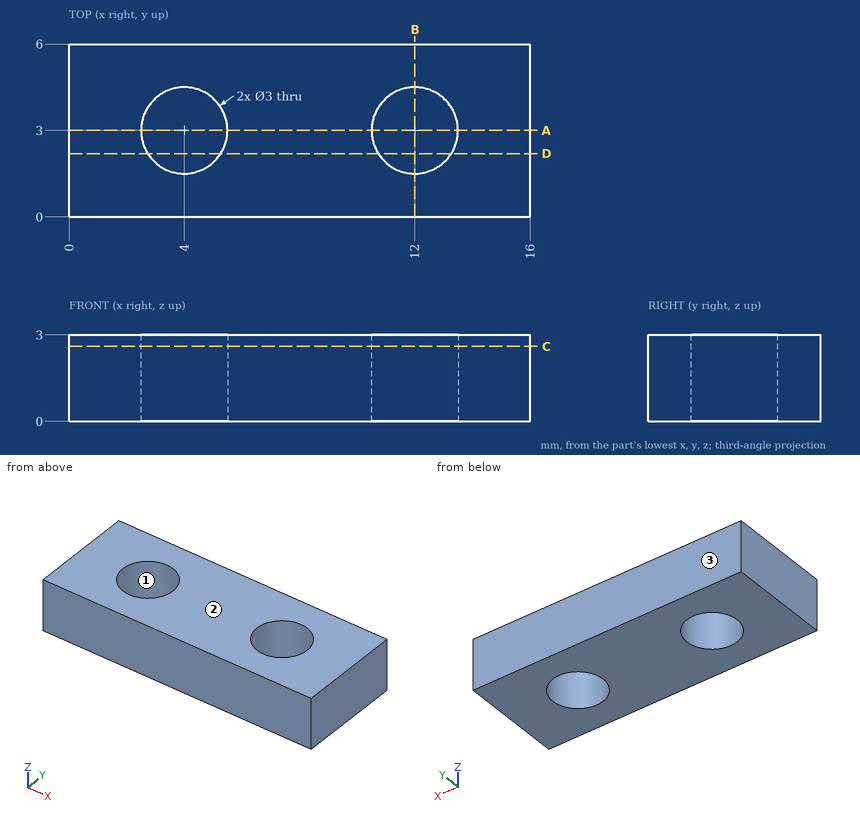
Job drawing, mm, ordinate dimensions from the low corner. One solid piece. Round coordinates to 2 decimals unless told otherwise and drop trailing zeros. Write each loop counter-clockwise with the first axis right and the second up, starting at its lowest first coordinate (ties: lowest second). Pieces come first, ordered by that corner, then holes.
1) Band-saw the part on A-A, the plane y = 3. List the corners of the cut face in (x, z).
2) Band-saw the part on D-D, the plane y = 2.2. List the corners of the cut face in (x, z).
3) Drill centre lines: probe 1 along Y at (x, z) = (4, 0.9); probe 2 along X at (y, z) = (1.75, 1.95); probe 3 along X at (y, z) = (2, 2.8). Where is each one in solid material? Low to high.
4) Mould opens along Y. For the marked faces 1, 2 and 3 say: +Y half, -Y half, draft (parallel to the pull), parting line (faces both ways), or undercut.
5) Band-saw the part on B-B, the plane x = 12. List the corners of the cut face in (y, z).
6) Band-saw the part on C-C, the plane z = 2.6. List the corners of the cut face in (x, y), and give its area (3 significant figures).
Ans:
1. outline: (0, 0) - (2.5, 0) - (2.5, 3) - (0, 3) - close; (5.5, 0) - (10.5, 0) - (10.5, 3) - (5.5, 3) - close; (13.5, 0) - (16, 0) - (16, 3) - (13.5, 3) - close
2. outline: (0, 0) - (2.73, 0) - (2.73, 3) - (0, 3) - close; (5.27, 0) - (10.73, 0) - (10.73, 3) - (5.27, 3) - close; (13.27, 0) - (16, 0) - (16, 3) - (13.27, 3) - close
3. probe 1: y = 0 to 1.5, 4.5 to 6
3. probe 2: x = 0 to 3.17, 4.83 to 11.17, 12.83 to 16
3. probe 3: x = 0 to 2.88, 5.12 to 10.88, 13.12 to 16
4. face 1: undercut
4. face 2: draft
4. face 3: +Y half
5. outline: (0, 0) - (1.5, 0) - (1.5, 3) - (0, 3) - close; (4.5, 0) - (6, 0) - (6, 3) - (4.5, 3) - close
6. outline: (0, 0) - (16, 0) - (16, 6) - (0, 6) - close; hole circle Ø3 at (4, 3); hole circle Ø3 at (12, 3)
6. area: 81.9 mm2
